Can you work these out from the model? Positions are in its coordinate system, mm. Face numbers are marked on the shaded views. A direction names the side the tool comes from. Give positions to 0.01 mm unless a question says otherwise; leave off trailing zeros. Write each loop counter-clockwise with the first axis right and the second up, starting at its lowest first coordinate (ties: lowest second). Pieces come first, ordered by that corner, then holes.
1. If I drill on probe 1 along X at (y, z) = (1.5, 5.25); probe 2 along X at (y, z) = (1, 5); probe 3 along Y at (x, z) = (3.5, 16.5), over which ranges is the centre line in solid material (lowest first)?
2. Suppose I cut it at B-B (x = -11). Please give me the cut outline in (y, z).
3. I'm going to push flat-ended pins straight in: pin 1 (5 mm diameter, centred on x = -3.5, z = -12.5, fed in from +Y); pin 2 (6 mm diameter, centred on x = -3.5, z = -9.5, fed in from -Y); pin 3 (5 mm diameter, centred on y = 0, z = -8.5, fed in from -X); pin 4 (6 mm diameter, centred on x = -9.09, z = 5.25, fed in from +Y). Where does each tip first touch, or does it pass through?
4. On a 3-axis mill with a long thin cutter (end or side, diameter ignored), from which of +Z, -Z, +X, -X, +Y, -Y can I reach the whole of each face in a straight line? I mean the marked faces 1 and 2. Say none if no direction works.
5. Thinking about a two-plate mould opening in Z: for the marked faces 3, 4, 5 and 6, which applies, pulls with the +Z half, pulls with the -Z half, needs draft (parallel to the pull), parting line crosses it, or undercut?
6. Suppose I cut it at A-A (z = -9.5). Please give me the cut outline in (x, y).
7. Suppose I cut it at D-D (y = -4). Please give me the cut outline in (x, z), and give its area (3 significant figures).
8. Suppose I cut it at C-C (z = 4). Please give me the cut outline in (x, y), and give its area (3 significant figures).
```python
from build123d import *

# Parameters (mm, degrees)
SKETCH_1_R               = 18.5
EXTRUDE_1_DEPTH          = 3
SKETCH_2_R               = 2.5
EXTRUDE_2_DEPTH          = 19.6
EXTRUDE_START            = 13
SKETCH_3_R               = 2.5
EXTRUDE_3_DEPTH          = 13
CUT_EXTRUDE_1_REACH      = 36.573
SKETCH_4_R               = 5
PATTERN_CIRCULAR_1_COUNT = 3


with BuildPart() as part:
    # 草图1 → 凸台-拉伸1 (new body)
    with BuildSketch(Plane(origin=(0, 0, 0), x_dir=(1, 0, 0), z_dir=(0, 1, 0))):
        with Locations(Location((0, 0, 0), (0, 0, 270))):
            Circle(SKETCH_1_R)
    extrude(amount=EXTRUDE_1_DEPTH)

    # 草图2 → 凸台-拉伸2 (add)
    with BuildSketch(Plane(origin=(0, 3, 0), x_dir=(1, 0, 0), z_dir=(0, 1, 0))):
        with Locations(Location((0, 0, 0), (0, 0, 270))):
            Circle(SKETCH_2_R)
    extrude(amount=EXTRUDE_2_DEPTH)

    # 草图3 → 凸台-拉伸3 (add)
    with BuildSketch(Plane(origin=(0, 0, 0), x_dir=(-1, 0, 0), z_dir=(0, -1, 0)).offset(EXTRUDE_START)):
        with Locations(Location((0, 0, 0), (0, 0, 270))):
            Circle(SKETCH_3_R)
    extrude(amount=-EXTRUDE_3_DEPTH)

    # 草图4 → 切除-拉伸1 (cut, up to next)
    with BuildSketch(Plane(origin=(0, 0, 0), x_dir=(-1, 0, 0), z_dir=(0, -1, 0)), mode=Mode.PRIVATE) as cut_extrude_1_sk1:
        with Locations(Location((0, 10.5, 0), (0, 0, 90))):
            Circle(SKETCH_4_R)
    cut_extrude_1_tool1 = extrude(cut_extrude_1_sk1.sketch, amount=-CUT_EXTRUDE_1_REACH, mode=Mode.PRIVATE) & part.part
    cut_extrude_1 = cut_extrude_1_tool1.solids().sort_by_distance((0, 0, -10.5))[0]
    add(cut_extrude_1, mode=Mode.SUBTRACT)

    # 阵列(圆周)1: 切除-拉伸1 ×3 about axis
    pattern_circular_1_axis = Axis((0, 0, 0), (0, 1, 0))
    for i in range(1, PATTERN_CIRCULAR_1_COUNT):
        add(cut_extrude_1.rotate(pattern_circular_1_axis, i * 360 / PATTERN_CIRCULAR_1_COUNT), mode=Mode.SUBTRACT)


solid = part.part
```
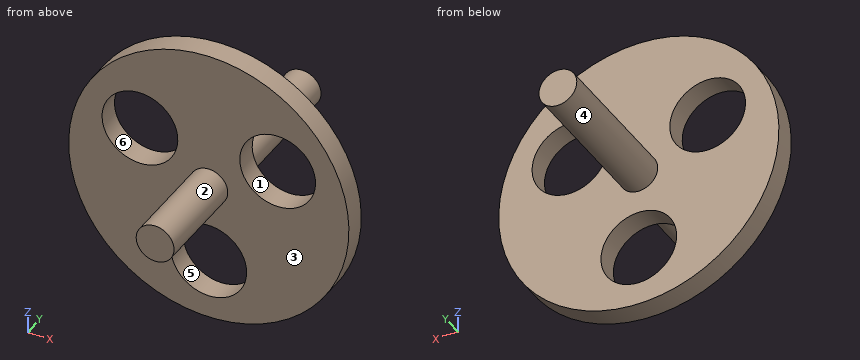
Checks:
1. probe 1: x = -17.74 to -14.09, -4.09 to 4.09, 14.09 to 17.74
1. probe 2: x = -17.81 to -14.09, -4.1 to 4.1, 14.09 to 17.81
1. probe 3: y = 0 to 3
2. outline: (0, -14.87) - (3, -14.87) - (3, 0.63) - (0, 0.63) - close; (0, 9.87) - (3, 9.87) - (3, 14.87) - (0, 14.87) - close
3. pin 1: stops at y = 3
3. pin 2: stops at y = 0
3. pin 3: stops at x = -17.5
3. pin 4: passes through
4. face 1: +Y, -Y
4. face 2: -Y
5. face 3: needs draft
5. face 4: parting line crosses it
5. face 5: undercut
5. face 6: undercut
6. outline: (-15.87, 0) - (-4.9, 0) - (-4.9, 3) - (-15.87, 3) - close; (4.9, 0) - (15.87, 0) - (15.87, 3) - (4.9, 3) - close
7. outline: circle Ø5 at (0, 0)
7. area: 19.6 mm2
8. outline: (-18.06, 0) - (-13.93, 0) - (-13.93, 3) - (-18.06, 3) - close; (-4.25, 0) - (4.25, 0) - (4.25, 3) - (-4.25, 3) - close; (13.93, 0) - (18.06, 0) - (18.06, 3) - (13.93, 3) - close
8. area: 50.3 mm2
